from build123d import *

# Parameters (mm, degrees)
SKETCH1_W           = 16
SKETCH1_H           = 14
BOSS_EXTRUDE1_DEPTH = 3


with BuildPart() as part:
    # Sketch1 → Boss-Extrude1 (new body)
    with BuildSketch(Plane(origin=(0, 0, 0), x_dir=(1, 0, 0), z_dir=(0, 1, 0))):
        with Locations((-34.802547771, 15.318471338)):
            Rectangle(SKETCH1_W, SKETCH1_H)
        with BuildLine():
            Line((-34.802547771, 21.085939893), (-37.354294581, 13.665043558))
            ThreePointArc((-37.354294581, 13.665043558), (-34.802547771, 11.113296747), (-32.250800961, 13.665043558))
            Line((-32.250800961, 13.665043558), (-34.802547771, 21.085939893))
        make_face(mode=Mode.SUBTRACT)
        Polygon((-39.65867818, 17.46662554), (-39.999163851, 16.697953343), (-40.947570701, 16.633402092), (-40.219675658, 16.200131233), (-40.517939861, 15.5267772), (-39.817900069, 15.960979096), (-38.76035915, 15.331490454), (-39.189256036, 16.350897547), (-38.460919473, 16.802650605), (-39.353755451, 16.741881664), align=None, mode=Mode.SUBTRACT)
        Polygon((-29.764149732, 12.454265734), (-30.098857658, 11.698637236), (-31.248127998, 11.913183956), (-30.492306767, 10.810396065), (-30.906618006, 9.875057055), (-30.188552158, 10.36720012), (-29.391182209, 9.203790192), (-29.573076572, 10.789030573), (-28.642568323, 11.42677596), (-29.668222777, 11.618245966), align=None, mode=Mode.SUBTRACT)
        Polygon((-30.906618006, 18.234753406), (-31.083034427, 17.927114996), (-31.326443698, 17.965418816), (-31.197762972, 17.727049113), (-31.558988429, 17.097137085), (-31.066185401, 17.48331326), (-30.857713309, 17.097137085), (-30.880567513, 17.628769359), (-30.59737318, 17.850689473), (-30.892101379, 17.897069037), align=None, mode=Mode.SUBTRACT)
    extrude(amount=BOSS_EXTRUDE1_DEPTH)


solid = part.part
Could you check a few things on this model? Use its own coordinates, in mm. A direction names the side the tool comes from. Round coordinates to 2 decimals unless told otherwise and drop trailing zeros. Loops run counter-clockwise (first coordinate to the right, second up) from the corner with the lowest first, then second, coordinate; pieces in that order, holes last. Notation, with made-up numbers: (3.25, -34.5) -> (21.25, -34.5) arc R18 cw to (21.25, -18.5) -> close; hole circle Ø10 at (-36.5, 79). An arc over 180 degrees is marked (long way). Use CSV: the item, a comma, the result in double quotes.
(1) If I drill on probe 1 along Z at (x, y) = (-31, 0.7); probe 2 along X at (y, z) = (0.3, -10.25); probe 3 along X at (y, z) = (2.3, -13.5), over which ranges is the centre line in solid material (lowest first)? Write a range as [from, to].
Return value:
probe 1,"z = [-22.32, -18.07], [-17.36, -11.87], [-11.55, -8.32]"
probe 2,"x = [-42.8, -30.74], [-30.36, -30.11], [-29.51, -26.8]"
probe 3,"x = [-42.8, -37.35], [-32.26, -26.8]"
(2) Suppose I cut it at B-B on z = -12.25. Write out the boundary of the cut face in (x, y).
Return value:
outline,"(-42.8, 0) -> (-36.93, 0) -> (-36.93, 3) -> (-42.8, 3) -> close; (-32.68, 0) -> (-29.85, 0) -> (-29.85, 3) -> (-32.68, 3) -> close; (-29.74, 0) -> (-26.8, 0) -> (-26.8, 3) -> (-29.74, 3) -> close"
(3) If we mould it in two halves opening along Z, with no side actions, what happens to faces 1 (the flat face through (-35, 1, -22.318)), 2 (the flat face through (-29.8, 1.5, -9.8)), 3 (the flat face through (-26.803, 1, -15))? For each: +Z half, -Z half, draft (parallel to the pull), parting line (faces both ways), or undercut.
Return value:
face 1,"-Z half"
face 2,"undercut"
face 3,"draft"
(4) Suppose I cut it at D-D on y = 1.9. Give the number of separate pieces and of enclosed holes in the cut face, plus the area to 3 significant figures.
Return value:
separate pieces,"1"
enclosed holes,"4"
area,"190 mm²"
(5) For faces 4 (the flat face through (-36.06, 1.48, -17.43)), 5 (the flat face through (-35, 1, -8.318)), which set-ups out of +Z, -Z, +X, -X, +Y, -Y let a thin tool reach every point of the face, with its end or its side?
Return value:
face 4,"+Y, -Y"
face 5,"+Z, +X, -X, +Y, -Y"
(6) Suppose I cut it at C-C on z = -14.5. Write out the boundary of the cut face in (x, y).
Return value:
outline,"(-42.8, 0) -> (-37.07, 0) -> (-37.07, 3) -> (-42.8, 3) -> close; (-32.54, 0) -> (-26.8, 0) -> (-26.8, 3) -> (-32.54, 3) -> close"
(7) Suppose I cut it at A-A on x = -33. Write out the boundary of the cut face in (y, z), plus the area to 3 significant figures.
Return value:
outline,"(0, -22.32) -> (3, -22.32) -> (3, -15.84) -> (0, -15.84) -> close; (0, -11.86) -> (3, -11.86) -> (3, -8.32) -> (0, -8.32) -> close"
area,"30.0 mm²"
